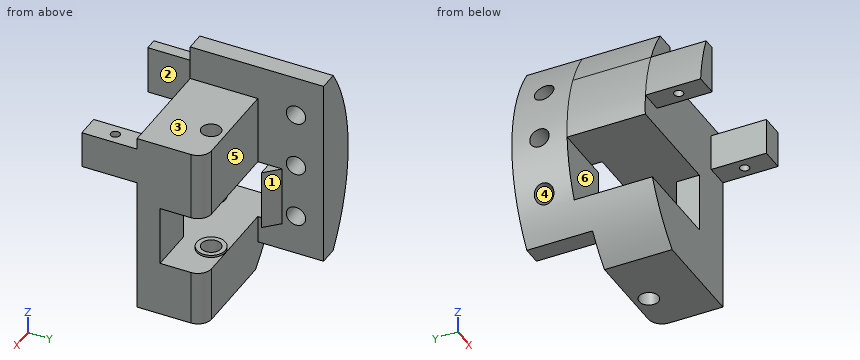
```python
from build123d import *
from build123d.topology import SkipClean

# Parameters (mm, degrees)
BOSS_EXTRUDE1_DEPTH       = 12
SKETCH1_W                 = 5
SKETCH1_H                 = 8
BOSS_EXTRUDE1_2_DEPTH     = 12
BOSS_EXTRUDE2_DEPTH       = 17
F_2_0MM_DOWEL_HOLE1_D     = 2
F_2_0MM_DOWEL_HOLE1_DEPTH = 8
BOSS_EXTRUDE6_START       = -17
BOSS_EXTRUDE6_DEPTH       = 17
BOSS_EXTRUDE8_DEPTH       = 12
CUT_EXTRUDE2_REACH        = 70.191
SKETCH5_R                 = 2.1
CUT_EXTRUDE3_REACH        = 70.191
SKETCH19_W                = 22.567285658
SKETCH19_H                = 2.3
CUT_EXTRUDE5_START        = -2.3
CUT_EXTRUDE5_DEPTH        = 2.3
SKETCH21_W                = 10
SKETCH21_H                = 13
BOSS_EXTRUDE10_DEPTH      = 5
FILLET3_R                 = 3
SKETCH23_R                = 3.1
SKETCH23_R_2              = 2.1
BOSS_EXTRUDE11_DEPTH      = 0.5
CUT_EXTRUDE6_START        = -1.5
SKETCH24_W                = 5
SKETCH24_H                = 12
SKETCH24_R                = 1
CUT_EXTRUDE6_DEPTH        = 1.5
BOSS_EXTRUDE12_START      = -9.5
SKETCH24_2_W              = 5
SKETCH24_2_H              = 12
SKETCH24_2_R              = 1
BOSS_EXTRUDE12_DEPTH      = 1.5
F_2_0MM_DOWEL_HOLE2_D     = 4.2
BOSS_EXTRUDE13_START      = 17
BOSS_EXTRUDE13_DEPTH      = 17
BOSS_EXTRUDE14_DEPTH      = 13


with BuildPart() as part:
    # Sketch1 → Boss-Extrude1 (new body)
    with BuildSketch(Plane(origin=(0, 0, 0), x_dir=(1, 0, 0), z_dir=(0, 1, 0))):
        with BuildLine():
            Line((-31.978879107, -1.25), (-36.978879107, -1.25))
            ThreePointArc((-36.978879107, -1.25), (-36.262349279, -7.351328095), (-34.546164765, -13.25))
            Line((-34.546164765, -13.25), (-31.978879107, -13.25))
            Line((-31.978879107, -13.25), (-31.978879107, -1.25))
        make_face()
    extrude(amount=BOSS_EXTRUDE1_DEPTH)



with BuildPart() as body_2:
    # Sketch1 → Boss-Extrude1 2 (new body)
    with BuildSketch(Plane(origin=(0, 0, 0), x_dir=(1, 0, 0), z_dir=(0, 1, 0))):
        with Locations((-6.478879107, -5.25)):
            Rectangle(SKETCH1_W, SKETCH1_H)
    extrude(amount=BOSS_EXTRUDE1_2_DEPTH)


with BuildPart() as part_1:
    add(part.part)

    add(body_2.part)  # Boss-Extrude2 merges body 2
    # Sketch2 → Boss-Extrude2 (add)
    with BuildSketch(Plane(origin=(0, 12, 0), x_dir=(1, 0, 0), z_dir=(0, 1, 0))):
        with BuildLine():
            Line((-3.978879107, -13.25), (-3.978879107, 1.75))
            Line((-3.978879107, 1.75), (-36.958591694, 1.75))
            ThreePointArc((-36.958591694, 1.75), (-36.530570062, -5.875155396), (-34.546164765, -13.25))
            Line((-34.546164765, -13.25), (-3.978879107, -13.25))
        make_face()
    extrude(amount=BOSS_EXTRUDE2_DEPTH)

    # Ø2.0mm Dowel Hole1
    with Locations(Plane(origin=(0, 0, 1.25), x_dir=(-1, 0, 0), z_dir=(0, 0, -1))):
        with Locations((6.478879107, 6), (34.478879107, 6)):
            Hole(F_2_0MM_DOWEL_HOLE1_D / 2, depth=F_2_0MM_DOWEL_HOLE1_DEPTH)



with BuildPart() as body_2_2:
    # Sketch13 → Boss-Extrude6 (new body)
    with BuildSketch(Plane(origin=(0, 29, 0), x_dir=(1, 0, 0), z_dir=(0, 1, 0)).offset(BOSS_EXTRUDE6_START)):
        with BuildLine():
            Line((-33.932838078, 14.75), (-24.958591694, 14.75))
            Line((-24.958591694, 14.75), (-3.978879107, 14.75))
            Line((-3.978879107, 14.75), (-3.978879107, 26.75))
            Line((-3.978879107, 26.75), (-25.562423594, 26.75))
            ThreePointArc((-25.562423594, 26.75), (-30.346689117, 21.167863843), (-33.932838078, 14.75))
        make_face()
    extrude(amount=BOSS_EXTRUDE6_DEPTH)


with BuildPart() as part_2:
    add(part_1.part)

    add(body_2_2.part)  # Boss-Extrude8 merges body 2 2
    # Sketch17 → Boss-Extrude8 (add)
    with BuildSketch(Plane(origin=(0, 29, 0), x_dir=(1, 0, 0), z_dir=(0, 1, 0))):
        with BuildLine():
            Line((-26.546164765, -20.75), (-26.546164765, 20.75))
            Line((-26.546164765, 20.75), (-30.63392727, 20.75))
            ThreePointArc((-30.63392727, 20.75), (-37, 0), (-30.63392727, -20.75))
            Line((-30.63392727, -20.75), (-26.546164765, -20.75))
        make_face()
    extrude(amount=BOSS_EXTRUDE8_DEPTH)

    # Cut-Extrude2: up to this face of the body (flat: up to its plane)
    cut_extrude2_end = Plane(part_2.part.faces().sort_by_distance((-14.77065135, 20.5, -26.75))[0])
    # Sketch5 → Cut-Extrude2 (cut, up to the picked face)
    with BuildSketch(Plane.XY.offset(13.25), mode=Mode.PRIVATE) as cut_extrude2_sk1:
        with Locations((-12.978879107, 23.5)):
            Circle(SKETCH5_R)
    cut_extrude2_tool1 = split(extrude(cut_extrude2_sk1.sketch, amount=-CUT_EXTRUDE2_REACH, mode=Mode.PRIVATE), bisect_by=cut_extrude2_end, keep=Keep.BOTH, mode=Mode.PRIVATE)
    add(cut_extrude2_tool1.solids().sort_by(Axis((-12.978879, 23.5, 13.25), (0, 0, -1)))[0], mode=Mode.SUBTRACT)

    # Cut-Extrude3: up to this face of the body (flat: up to its plane)
    cut_extrude3_end = Plane(part_2.part.faces().sort_by_distance((-14.840961104, 20.382278978, -26.75))[0])
    # Sketch19 → Cut-Extrude3 (cut, up to the picked face)
    with BuildSketch(Plane.XY.offset(13.25), mode=Mode.PRIVATE) as cut_extrude3_sk1:
        with Locations((-15.262521936, 27.85)):
            Rectangle(SKETCH19_W, SKETCH19_H)
    cut_extrude3_tool1 = split(extrude(cut_extrude3_sk1.sketch, amount=-CUT_EXTRUDE3_REACH, mode=Mode.PRIVATE), bisect_by=cut_extrude3_end, keep=Keep.BOTH, mode=Mode.PRIVATE)
    add(cut_extrude3_tool1.solids().sort_by(Axis((-15.262522, 27.85, 13.25), (0, 0, -1)))[0], mode=Mode.SUBTRACT)

    # Sketch22 → Cut-Extrude5 (cut)
    with BuildSketch(Plane(origin=(0, 29, 0), x_dir=(1, 0, 0), z_dir=(0, 1, 0)).offset(CUT_EXTRUDE5_START)):
        with BuildLine():
            Line((-26.546164765, 20.75), (-26.546164765, 25.774039968))
            ThreePointArc((-26.546164765, 25.774039968), (-28.700191214, 23.351638578), (-30.63392727, 20.75))
            Line((-30.63392727, 20.75), (-26.546164765, 20.75))
        make_face()
    extrude(amount=CUT_EXTRUDE5_DEPTH, mode=Mode.SUBTRACT)

    # Sketch21 → Boss-Extrude10 (add)
    with BuildSketch(Plane.XZ.offset(-12)):
        with Locations((-8.978879107, -8.25)):
            Rectangle(SKETCH21_W, SKETCH21_H)
    extrude(amount=-BOSS_EXTRUDE10_DEPTH)

    # Fillet3
    fillet3_edges = [part_2.edges().sort_by_distance(p)[0] for p in [
        (-3.978879107, 26.7, -20.75),
        (-3.978879107, 26.7, 5.75),
    ]]
    fillet(fillet3_edges, radius=FILLET3_R)

    # Sketch23 → Boss-Extrude11 (add)
    with BuildSketch(Plane(origin=(0, 0, -1.75), x_dir=(-1, 0, 0), z_dir=(0, 0, -1))):
        with Locations(Location((12.978879107, 23.5, 0), (0, 0, 180))):
            Circle(SKETCH23_R)
        with Locations(Location((12.978879107, 23.5, 0), (0, 0, 180))):
            Circle(SKETCH23_R_2, mode=Mode.SUBTRACT)
    boss_extrude11 = extrude(amount=BOSS_EXTRUDE11_DEPTH)

    # Mirror4: Boss-Extrude11 across plane
    add(boss_extrude11.mirror(Plane.XY.offset(-8.25)))

    # Sketch24 → Cut-Extrude6 (cut)
    # profile 1 of 2: a face of its own
    with BuildSketch(Plane(origin=(0, 0, 1.25), x_dir=(-1, 0, 0), z_dir=(0, 0, -1)).offset(CUT_EXTRUDE6_START)):
        with Locations((34.478879107, 6)):
            Rectangle(SKETCH24_W, SKETCH24_H)
        with Locations((34.478879107, 6)):
            Circle(SKETCH24_R, mode=Mode.SUBTRACT)
    # profile 2 of 2: a face of its own
    with BuildSketch(Plane(origin=(0, 0, 1.25), x_dir=(-1, 0, 0), z_dir=(0, 0, -1)).offset(CUT_EXTRUDE6_START)):
        with Locations((6.478879107, 6)):
            Rectangle(SKETCH24_W, SKETCH24_H)
        with Locations((6.478879107, 6)):
            Circle(SKETCH24_R, mode=Mode.SUBTRACT)
    extrude(amount=CUT_EXTRUDE6_DEPTH, mode=Mode.SUBTRACT)

    # Sketch24<2> → Boss-Extrude12 (add)
    with BuildSketch(Plane(origin=(0, 0, 1.25), x_dir=(-1, 0, 0), z_dir=(0, 0, -1)).offset(BOSS_EXTRUDE12_START)):
        with Locations((6.478879107, 6)):
            Rectangle(SKETCH24_2_W, SKETCH24_2_H)
        with Locations((6.478879107, 6)):
            Circle(SKETCH24_2_R, mode=Mode.SUBTRACT)
    extrude(amount=BOSS_EXTRUDE12_DEPTH)

    # Ø2.0mm Dowel Hole2 (through all)
    with Locations(Plane(origin=(-26.546164765, 0, 0), x_dir=(0, 0, -1), z_dir=(1, 0, 0))):
        with Locations((-12, 35), (0, 35), (12, 35)):
            Hole(F_2_0MM_DOWEL_HOLE2_D / 2)

    # Sketch27 → Boss-Extrude13 (add)
    with SkipClean():  # the faces are left unmerged after this step: merging them gives an invalid solid
        with BuildSketch(Plane.XZ.offset(-29).offset(BOSS_EXTRUDE13_START)):
            with BuildLine():
                Line((-34.546164765, 13.25), (-26.546164765, 13.25))
                Line((-26.546164765, 13.25), (-26.546164765, 20.75))
                Line((-26.546164765, 20.75), (-30.63392727, 20.75))
                ThreePointArc((-30.63392727, 20.75), (-32.805084963, 17.112171123), (-34.546164765, 13.25))
            make_face()
        extrude(amount=-BOSS_EXTRUDE13_DEPTH)

    # Sketch28 → Boss-Extrude14 (add)
    with SkipClean():  # the faces are left unmerged after this step: merging them gives an invalid solid
        with BuildSketch(Plane(origin=(0, 0, -1.75), x_dir=(-1, 0, 0), z_dir=(0, 0, -1))):
            Polygon((26.546164765, 29), (23.546164765, 29), (26.546164765, 32), align=None)
        extrude(amount=BOSS_EXTRUDE14_DEPTH)


solid = part_2.part
```
Source: CAD feature listing. Evaluate the final solid. Frame: model axes, mm. Face numbers are marked on the shaded views. A direction names the side the tool comes from. Give positions to 0.01 mm unless a question says otherwise; leave off trailing zeros. Loops run counter-clockwise (first coordinate to the right, second up) from the corner with the lowest first, then second, coordinate; pieces in that order, holes last. Notation, with made-up numbers: (-27.75, -12.75) -> (-17.75, -12.75) arc R30 ccw to (-17.75, 23.25) -> close; hole circle Ø10 at (36.25, 23.25). An arc over 180 degrees is marked (long way). Use a Markdown table: item, result. Add a question column.
(1) Ray query, line 1 (Z direction, x = -28.75, y = 35); line 2 (Z direction, x = -32, y = 35); line 3 (Y direction, x = -28, z = -12). Return the intervals inside material, ascending.
(2) Section query B-B (x = -20). Output: boundary loops of the cut face in (y, z).
(3) Section query C-C (y = 6). Output: boundary loops of the cut face in (x, z).
(4) Section query D-D (x = -12.5). Output: boundary loops of the cut face in (y, z).
(5) First-contact query: pin 1 Ø16.5 at (x, z) = (-21.5, 6.5) entering from -Y; pin 2 Ø3.5 at (x, y) = (-25, 31) entering from -Z; pin 3 Ø4 at (x, y) = (-6, 6) entering from -Z. Flat tips, straight axial feed; report the tip coordinate or a pass-through.
(6) Pull-direction query (Y, two-part tool) for the marked faces 3, 4, 5 and 6; classes: +Y half, -Y half, draft (parallel to the pull), parting line (faces both ways), or undercut.
(7) Access query for the marked faces 1 and 2. Directions: +Z, -Z, +X, -X, +Y, -Y. A direction counts if a zero-diameter tool reaches every point of the face in a straight line with its end or side. Return the directions, or none.
(8) Section query A-A (z = 12). Output: boundary loops of the cut face in (x, y).
Checked values:
| question | item | result |
|---|---|---|
| 1 | line 1 | -20.75 to -14.1, -9.9 to -2.1, 2.1 to 9.9, 14.1 to 20.75 |
| 1 | line 2 | -18.57 to -14.1, -9.9 to -2.1, 2.1 to 9.9, 14.1 to 18.57 |
| 1 | line 3 | 29 to 32.9, 37.1 to 41 |
| 2 | outline | (12, -26.75) -> (26.7, -26.75) -> (26.7, -14.75) -> (12, -14.75) -> close; (12, -1.75) -> (26.7, -1.75) -> (26.7, 13.25) -> (12, 13.25) -> close |
| 3 | outline | (-36.9, 2.75) -> (-35.48, 2.75) -> (-35.48, 9.25) -> (-33.48, 9.25) -> (-33.48, 2.75) -> (-31.98, 2.75) -> (-31.98, 13.25) -> (-34.55, 13.25) arc R37 ccw to start; (-8.98, 2.75) -> (-7.48, 2.75) -> (-7.48, 10.75) -> (-8.98, 10.75) -> close; (-5.48, 2.75) -> (-3.98, 2.75) -> (-3.98, 10.75) -> (-5.48, 10.75) -> close |
| 4 | outline | (12, -26.75) -> (21.46, -26.75) -> (21.46, -14.25) -> (20.44, -14.25) -> (20.44, -14.75) -> (17, -14.75) -> (17, -1.75) -> (20.44, -1.75) -> (20.44, -2.25) -> (21.46, -2.25) -> (21.46, 13.25) -> (12, 13.25) -> close; (25.54, -26.75) -> (26.7, -26.75) -> (26.7, -14.75) -> (26.56, -14.75) -> (26.56, -14.25) -> (25.54, -14.25) -> close; (25.54, -2.25) -> (26.56, -2.25) -> (26.56, -1.75) -> (26.7, -1.75) -> (26.7, 13.25) -> (25.54, 13.25) -> close |
| 5 | pin 1 | y = 12 |
| 5 | pin 2 | z = -20.75 |
| 5 | pin 3 | z = 2.75 |
| 6 | face 3 | draft |
| 6 | face 4 | undercut |
| 6 | face 5 | +Y half |
| 6 | face 6 | -Y half |
| 7 | face 1 | +Z, -Z, +X, +Y |
| 7 | face 2 | +Z, -Z, -Y |
| 8 | outline | (-35, 0) -> (-31.98, 0) -> (-31.98, 12) -> (-3.98, 12) -> (-3.98, 23.7) arc R3 ccw to (-6.98, 26.7) -> (-26.55, 26.7) -> (-26.55, 32.9) -> (-35, 32.9) -> close; (-35, 37.1) -> (-26.55, 37.1) -> (-26.55, 41) -> (-35, 41) -> close; hole circle Ø4.2 at (-12.98, 23.5) |
